Geometry: final body of the model. Coordinates: model frame, mm. A direction names the side the tool comes from. Give positions to 0.01 mm unless a question says otherwise; leave off trailing zeros. Loops run counter-clockwise (first coordinate to the right, second up) from the corner with the lowest first, then second, coordinate; pieces in that order, holes last. Notation, with made-up numbers: (57.5, -25.5) - (98.5, -25.5) arc R31 ccw to (98.5, 7.5) - close; hole circle Ø1 at (22, 33.25). An arc over 180 degrees is marked (long way). Use one line per item in the form item = value.
```python
from build123d import *

# Parameters (mm, degrees)
SKETCH_1_W      = 30
SKETCH_1_H      = 20
EXTRUDE_1_DEPTH = 460
SKETCH_2_W      = 20
SKETCH_2_H      = 10
EXTRUDE_2_DEPTH = 460


with BuildPart() as part:
    # 草图1 → 凸台-拉伸1 (new body)
    with BuildSketch(Plane(origin=(0, 0, 0), x_dir=(1, 0, 0), z_dir=(0, 1, 0))):
        with Locations((-15, 10)):
            Rectangle(SKETCH_1_W, SKETCH_1_H)
    extrude(amount=EXTRUDE_1_DEPTH)

    # 草图2 → 凸台-拉伸2 (add)
    with BuildSketch(Plane.ZY.offset(30)):
        with Locations((-10, 455)):
            Rectangle(SKETCH_2_W, SKETCH_2_H)
    extrude(amount=EXTRUDE_2_DEPTH)


solid = part.part
```
(1) Pin query (flat end, axial travel): P1, Ø6, axis at y = 161, z = -8, coming from the -X side; P2, Ø6, axis at x = -197, z = -3, coming from the -Y side. Return the tip coordinate at first contact, or that it passes through.
Solution:
P1 = -30
P2 = 450
(2) Cut plane A-A (x = -272). Return the cut outline in (y, z), plus the area to 3 significant figures.
Solution:
outline = (450, -20) - (460, -20) - (460, 0) - (450, 0) - close
area = 200 mm2
(3) Cut plane B-B (z = -10.75). Return the cut outline in (x, y), plus the area to 3 significant figures.
Solution:
outline = (-490, 450) - (-30, 450) - (-30, 0) - (0, 0) - (0, 460) - (-490, 460) - close
area = 18,400 mm2
(4) Access query for faces 1 (the face through (-26, 297, 0)), 2 (the face through (-30, 222, -10)). Directions: +Z, -Z, +X, -X, +Y, -Y. A direction counts if a zero-diameter tool reaches every point of the face in a straight line with its end or side. Return the directions, or none.
Solution:
face_1 = +Z, +X, -X, +Y, -Y
face_2 = +Z, -Z, -X, -Y
(5) Cut plane C-C (y = 260). Return the cut outline in (x, z), plus the area to 3 significant figures.
Solution:
outline = (-30, -20) - (0, -20) - (0, 0) - (-30, 0) - close
area = 600 mm2
(6) Material intervals for L1, parallel to X at y = 412, z = -10; L2, parallel to Y at x = -156, z = -16.75, sorted ascending. Write a range as from..to.
Solution:
L1 = -30..0
L2 = 450..460
